Geometry check sheet. Reference: the model listing, model coordinates, mm. A direction names the side the tool comes from. Give positions to 0.01 mm unless a question says otherwise; leave off trailing zeros. Write each loop counter-clockwise with the first axis right and the second up, starting at its lowest first coordinate (ties: lowest second). Pieces come first, ordered by that corner, then holes. Notation, with made-up numbers: (27.25, 55.5) - (68.25, 55.5) arc R36 cw to (68.25, 90.5) - close; hole circle Ø6 at (88.5, 20.5). An arc over 180 degrees is marked (long way). Write item = value, one per line. Start each with the question number.
(1) Draft check along X on faces 1 (the flat face through (-38.227, -20, 3)), 2 (the flat face through (22.225, 66, 3)), 3 (the cylindrical face through (27.22, 58.1, 3.13)), 4 (the flat face through (-35, -32.507, 3)). Enter one of: pulls with the +X half, pulls with the -X half, needs draft (parallel to the pull), parting line crosses it, or undercut.
(2) Section check B-B, the plane y = 38. Enter the section's corners in (x, z), plus the area to 3 significant figures.
(3) Access from +Z, -Z, +X, -X, +Y, -Y to the whole of each face (thin tool, end or side, straight path). Record for faces 5 (the cylindrical face through (-27.15, -60.68, 3.13)), 6 (the flat face through (-31, -11, 6.35)), 7 (the flat face through (32.639, -1, 3)), 8 (the flat face through (-32.639, -1, 3)).
(4) Section check A-A, the plane x = -6.5. Enter the section's corners in (y, z).
(5) Thickness scan on L1, parallel to Y at x = -33, z = 2.75; L2, parallel to Y at x = 19.5, z = 0.75; L3, parallel to X at y = 38, z = 4. Record the ranges inside material, lowest first.
(6) Depth check by flat-ended pin: pin 1 Ø1.7 at (x, z) = (36.5, 4) entering from -Y; pin 2 Ø4 at (x, y) = (-28, 44) entering from +Z; pin 3 Ø1.9 at (y, z) = (-47.5, 2.5) entering from +X; pin 4 Ø3 at (y, z) = (-3, 3.5) entering from +X. Enter the tip coordinate at first touch or a pass-through.
```python
from build123d import *

# Parameters (mm, degrees)
F1_DEPTH = 6.35


with BuildPart() as f1:
    # F0 (on Top) → F1 (new body)
    with BuildSketch(Plane.XY):
        with BuildLine():
            Line((-22.225, 69.092832), (-32.639, 69.092832))
            ThreePointArc((-32.639, 69.092832), (-36.590313, 67.456144), (-38.227, 63.504832))
            Line((-38.227, 63.504832), (-38.227, 43.692832))
            Line((-38.227, 43.692832), (-32.639, 43.692832))
            Line((-32.639, 43.692832), (-32.639, 30.775996))
            Line((-32.639, 30.775996), (-38.227, 30.992832))
            Line((-38.227, 30.992832), (-38.227, 5.592832))
            Line((-38.227, 5.592832), (-32.639, 5.592832))
            Line((-32.639, 5.592832), (-32.639, -7.107168))
            Line((-32.639, -7.107168), (-38.227, -7.107168))
            Line((-38.227, -7.107168), (-38.227, -32.507168))
            Line((-38.227, -32.507168), (-32.639, -32.507168))
            Line((-32.639, -32.507168), (-32.639, -45.207168))
            Line((-32.639, -45.207168), (-38.227, -45.207168))
            Line((-38.227, -45.207168), (-38.227, -52.56587))
            Line((-38.227, -52.56587), (-38.227, -66.085968))
            ThreePointArc((-38.227, -66.085968), (-36.590313, -70.037281), (-32.639, -71.673968))
            Line((-32.639, -71.673968), (-22.225, -71.673968))
            Line((-22.225, -71.673968), (-9.525, -71.673968))
            Line((-9.525, -71.673968), (9.525, -71.673968))
            Line((9.525, -71.673968), (22.225, -71.673968))
            Line((22.225, -71.673968), (32.706467, -71.673968))
            ThreePointArc((32.706467, -71.673968), (36.667636, -70.0274), (38.294397, -66.058055))
            Line((38.294397, -66.058055), (38.227, -52.56587))
            Line((38.227, -52.56587), (38.227, -45.207168))
            Line((38.227, -45.207168), (32.639, -45.207168))
            Line((32.639, -45.207168), (32.639, -32.507168))
            Line((32.639, -32.507168), (38.227, -32.507168))
            Line((38.227, -32.507168), (38.227, -7.107168))
            Line((38.227, -7.107168), (32.639, -7.107168))
            Line((32.639, -7.107168), (32.639, 5.592832))
            Line((32.639, 5.592832), (38.227, 5.592832))
            Line((38.227, 5.592832), (38.227, 30.992832))
            Line((38.227, 30.992832), (32.639, 30.992832))
            Line((32.639, 30.992832), (32.639, 43.692832))
            Line((32.639, 43.692832), (38.227, 43.692832))
            Line((38.227, 43.692832), (38.227, 63.504832))
            ThreePointArc((38.227, 63.504832), (36.590313, 67.456144), (32.639, 69.092832))
            Line((32.639, 69.092832), (22.225, 69.092832))
            Line((22.225, 69.092832), (22.225, 63.504832))
            Line((22.225, 63.504832), (9.525, 63.504832))
            Line((9.525, 63.504832), (9.525, 69.092832))
            Line((9.525, 69.092832), (-9.525, 69.092832))
            Line((-9.525, 69.092832), (-9.525, 63.504832))
            Line((-9.525, 63.504832), (-22.225, 63.504832))
            Line((-22.225, 63.504832), (-22.225, 69.092832))
        make_face()
        with BuildLine():
            Line((-28.829, -56.687968), (-28.829, 54.106832))
            ThreePointArc((-28.829, 54.106832), (-27.192313, 58.058144), (-23.241, 59.694832))
            Line((-23.241, 59.694832), (23.308467, 59.694832))
            ThreePointArc((23.308467, 59.694832), (27.25978, 58.058144), (28.896467, 54.106832))
            Line((28.896467, 54.106832), (28.896467, -56.687968))
            ThreePointArc((28.896467, -56.687968), (27.25978, -60.639281), (23.308467, -62.275968))
            Line((23.308467, -62.275968), (-23.241, -62.275968))
            ThreePointArc((-23.241, -62.275968), (-27.192313, -60.639281), (-28.829, -56.687968))
        make_face(mode=Mode.SUBTRACT)
    extrude(amount=F1_DEPTH)


solid = f1.part
```
Model answer:
q1.face_1 = pulls with the -X half
q1.face_2 = undercut
q1.face_3 = undercut
q1.face_4 = needs draft
q2.outline = (-32.64, 0) - (-28.83, 0) - (-28.83, 6.35) - (-32.64, 6.35) - close; (28.9, 0) - (32.64, 0) - (32.64, 6.35) - (28.9, 6.35) - close
q2.area = 48.0 mm²
q3.face_5 = +Z, -Z
q3.face_6 = +Z, +X, -X, +Y, -Y
q3.face_7 = +Z, -Z, +X
q3.face_8 = +Z, -Z, -X
q4.outline = (-71.67, 0) - (-62.28, 0) - (-62.28, 6.35) - (-71.67, 6.35) - close; (59.69, 0) - (69.09, 0) - (69.09, 6.35) - (59.69, 6.35) - close
q5.L1 = -71.66 to -45.21, -32.51 to -7.11, 5.59 to 30.79, 43.69 to 69.08
q5.L2 = -71.67 to -62.28, 59.69 to 63.5
q5.L3 = -32.64 to -28.83, 28.9 to 32.64
q6.pin_1 = -70.84
q6.pin_2 = 6.35
q6.pin_3 = 38.23
q6.pin_4 = 32.64
